Input: part model. Units: mm. Frame: model coordinates. Face numbers are marked on the shaded views. Coordinates: 2 decimals unless noted, no trailing zeros. Order: outer loops, then holes, each group sorted by start corner. A loop starts at its lowest first (then second) coordinate and runs counter-clockwise, first axis right, second up. Notation, with made-up numbers: (54, 19) - (106, 19) arc R16 ccw to (106, 48) - close; hole circle Ø3 at (33.5, 21.25). An arc over 180 degrees is marked (long way). One line per question, with ' | ' between items.
Autodesk Inventor part; units mm, degrees
ref_plane "YZ Plane" through (0, 0, 0) normal (1, 0, 0) x (0, 1, 0)
ref_plane "XZ Plane" through (0, 0, 0) normal (0, 1, 0) x (-1, 0, 0)
ref_plane "XY Plane" through (0, 0, 0) normal (0, 0, 1) x (1, 0, 0)
sketch "Эскиз1" plane through (0, 0, 0) normal (0, 0, 1) x (1, 0, 0)
  line L0 (0, 3.5) -> (0, -3.5)
  line L1 (15, -3.2113) -> (15.5, -3.5)
  line L2 (15.5, -3.5) -> (24, 0.6457)
  line L3 (15, -3.2113) -> (15, 2.5)
  line L4 (0, -3.5) -> (15.5, -3.5) construction
  line L5 (24, 0.6457) -> (24, 3.5)
  line L6 (24, 3.5) -> (16, 3.5)
  line L7 (15, 2.5) -> (16, 3.5)
  point P0 (0, 0)
  point P1 (0, 0)
  point P2 (15, 3.5)
  dimension "d0" = 7
  dimension "d1" = 60
  dimension "d2" = 31
  dimension "d3" = 30
  dimension "d4" = 26
  dimension "d5" = 48
  dimension "d9" = 1
  dimension "d10" = 45
revolve "Вращение1" add sketch "Эскиз1" angle 360 about axis through (0, 3.5, 0) along (0, -1, 0)
sketch "Эскиз2" plane through (0, 3.5, 0) normal (0, 1, 0) x (1, 0, 0)
  circle A0 centre (0, 0) radius 24
  line L0 (3, 24) -> (-3, 24)
  line L1 (-3, 24) -> (-3, 21.5)
  line L2 (-3, 21.5) -> (3, 21.5)
  line L3 (3, 21.5) -> (3, 24)
  point P0 (0, 0)
  point P1 (0, 24)
  point P2 (3, 23.8118)
  point P3 (-3, 23.8118)
  dimension "d12" = 2.5
  dimension "d13" = 6
extrude "Выдавливание1" cut sketch "Эскиз2" against normal through all contours L3 L2 L1 A0 picked at (0, 22.3333)
pattern_circular "Круговой массив1" count 4 over 360 about axis through (0, -10, 0) along (0, 1, 0) of "Выдавливание1"
thread "Резьба1"
properties part number "69. Гайка стопорная"
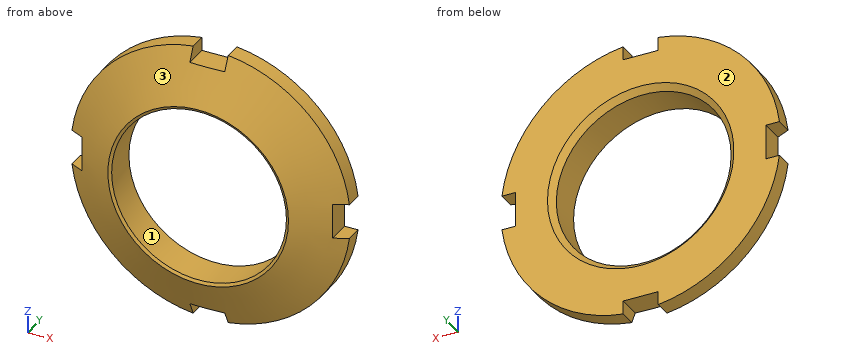
Item 1: Draft query along X for the marked faces 1, 2 and 3. Return one class per face: released by +X, released by -X, zero draft, split by the parting line, or undercut.
Data:
face 1: undercut | face 2: zero draft | face 3: split by the parting line
Item 2: Contact query for flat-ended pins moving along their axis: P1, Ø0.7, axis at x = 22.5, y = 2.5, coming from the +Z side; P2, Ø1, axis at y = 1, z = 18, coming from the +X side; P3, Ø2, axis at x = -1, y = 2, coming from the +Z side. Output: stop coordinate, or through.
Data:
P1: z = 9.24 | P2: x = 16.42 | P3: z = 21.5
Item 3: Section B-B on x = 0. Return the cut outline in (y, z), and give its area (3 significant figures).
Data:
outline: (-3.5, -15.5) - (-0.57, -21.5) - (3.5, -21.5) - (3.5, -16) - (2.5, -15) - (-3.21, -15) - close; (-3.5, 15.5) - (-3.21, 15) - (2.5, 15) - (3.5, 16) - (3.5, 21.5) - (-0.57, 21.5) - close | area: 72.3 mm^2
Item 4: Ray query, line 1 (Z direction, x = 0, y = 1.3); line 2 (Z direction, x = 9, y = 2.5); line 3 (X direction, y = 1.75, z = 1). Return the intervals inside material, ascending.
Data:
line 1: -21.5 to -15, 15 to 21.5 | line 2: -22.25 to -12, 12 to 22.25 | line 3: -21.5 to -14.97, 14.97 to 21.5
Item 5: Section A-A on z = 0. Return the cut outline in (x, y).
Data:
outline: (-21.5, -0.57) - (-15.5, -3.5) - (-15, -3.21) - (-15, 2.5) - (-16, 3.5) - (-21.5, 3.5) - close; (15, -3.21) - (15.5, -3.5) - (21.5, -0.57) - (21.5, 3.5) - (16, 3.5) - (15, 2.5) - close
Item 6: Section C-C on y = 1.25. Return the cut outline in (x, z).
Data:
outline: (-23.81, -3) arc R24 ccw to (-3, -23.81) - (-3, -21.5) - (3, -21.5) - (3, -23.81) arc R24 ccw to (23.81, -3) - (21.5, -3) - (21.5, 3) - (23.81, 3) arc R24 ccw to (3, 23.81) - (3, 21.5) - (-3, 21.5) - (-3, 23.81) arc R24 ccw to (-23.81, 3) - (-21.5, 3) - (-21.5, -3) - close; hole circle Ø30 at (0, 0)
